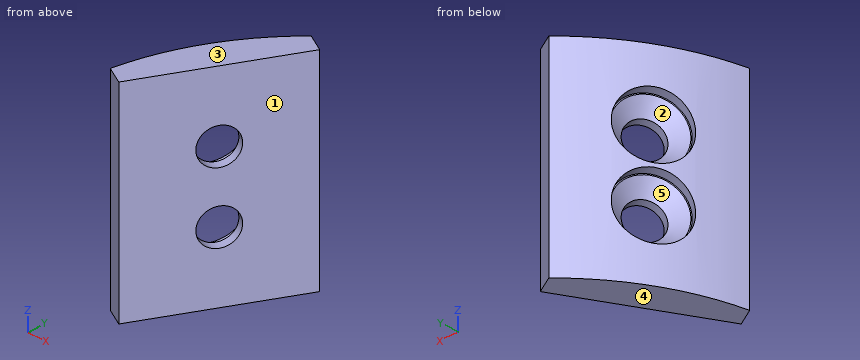
```python
from build123d import *

# Parameters (mm, degrees)
ESTRUSIONE_ESTRUSIONE1_DEPTH = 20
SCHIZZO3_R                   = 1.75
TAGLIO_ESTRUSIONE1_DEPTH     = 10.690610833
SCHIZZO3_3_R                 = 3.15
SCHIZZO3_3_R_2               = 1.75
TAGLIO_ESTRUSIONE2_DEPTH     = 1
SMUSSO2_SIZE                 = 1.3


with BuildPart() as part:
    # Schizzo2 → Estrusione-Estrusione1 (new body)
    with BuildSketch(Plane.XY):
        Polygon((-5.767949192, 11.990381057), (-7.5, 12.990381057), (-15, 0), (-13.267949192, -1), align=None)
        with BuildLine():
            Line((-15, 0), (-7.5, 12.990381057))
            ThreePointArc((-7.5, 12.990381057), (-12.285264352, 7.092900681), (-15, 0))
        make_face()
    extrude(amount=ESTRUSIONE_ESTRUSIONE1_DEPTH)

    # Schizzo3 → Taglio-Estrusione1 (cut, through all)
    with BuildSketch(Plane(origin=(-12.285264352, 7.092900681, 0), x_dir=(0, 0, 1), z_dir=(-0.866025404, 0.5, 0))):
        with Locations((6.666666667, 0)):
            Circle(SCHIZZO3_R)
        with Locations((13.333333333, 0)):
            Circle(SCHIZZO3_R)
    extrude(amount=-TAGLIO_ESTRUSIONE1_DEPTH, mode=Mode.SUBTRACT)

    # Schizzo3_3 → Taglio-Estrusione2 (cut)
    with BuildSketch(Plane(origin=(-12.285264352, 7.092900681, 0), x_dir=(0, 0, 1), z_dir=(-0.866025404, 0.5, 0))):
        with Locations((6.666666667, 0)):
            Circle(SCHIZZO3_3_R)
        with Locations((6.666666667, 0)):
            Circle(SCHIZZO3_3_R_2, mode=Mode.SUBTRACT)
        with Locations((13.333333333, 0)):
            Circle(SCHIZZO3_3_R)
        with Locations((13.333333333, 0)):
            Circle(SCHIZZO3_3_R_2, mode=Mode.SUBTRACT)
    extrude(amount=-TAGLIO_ESTRUSIONE2_DEPTH, mode=Mode.SUBTRACT)

    # Smusso2
    smusso2_edges = [part.edges().sort_by_distance(p)[0] for p in [
        (-11.419238948, 6.592900681, 4.916666667),
        (-11.419238948, 6.592900681, 11.583333333),
    ]]
    chamfer(smusso2_edges, length=SMUSSO2_SIZE)


solid = part.part
```
Here's how the part is built. I have some questions about the finished solid (model axes, mm). Face numbers are marked on the shaded views. A direction names the side the tool comes from. Give positions to 0.01 mm unless a question says otherwise; leave off trailing zeros. Order: outer loops, then holes, each group sorted by start corner. A loop starts at its lowest first (then second) coordinate and runs counter-clockwise, first axis right, second up. Notation, with made-up numbers: (16.25, 11.25) - (33.25, 11.25) arc R21 cw to (33.25, 25.25) - close; hole circle Ø9 at (-34.5, 9). An arc over 180 degrees is marked (long way). Answer as a JSON object with one key per item and string values. Group by question number.
Item 1: Please list where these lines run through material, in increasing order: probe 1 along Z at (x, y) = (-12, 7); probe 2 along Z at (x, y) = (-13.5, 4.5); probe 3 along X at (y, z) = (3.5, 5).
Item 2: If we mould it in two halves opening along Y, with no side actions, what happens to the marked faces 1, 2 and 3? For each: pulls with the +Y half, pulls with the -Y half, needs draft (parallel to the pull), parting line crosses it, or undercut.
Item 3: If we section it at A-A on z = 3: Please give me the cut outline in (x, y) (3 decimals), and give its area (3 significant figures).
Item 4: If we section it at B-B on x = -8.25: Please give me the cut outline in (y, z), and give its area (3 significant figures).
Item 5: For P1, Ø5, axis at x = -13, y = 4.5, coming from the -Z side; P2, Ø3, axis at y = 2.5, z = 2, coming from the +X side; P3, Ø3, axis at x = -8.5, z = 17.5, coming from the +Y side; P4, Ø4, axis at x = -14, z = 17.5, coming from the -Y side, each with a flat end and sliding along its axis, tell me the tip position at first contact or that it passes through.
Item 6: Which directions (+Z, -Z, +X, -X, +Y, -Y) give clear straight access to the entire face, cutting with the end or side of a thin tool? Please do the marked faces 4 and 5.
Result set:
{
 "1": {"probe 1": "0 to 3.52, 9.82 to 10.18, 16.48 to 20", "probe 2": "0 to 5.33, 8 to 12, 14.67 to 20", "probe 3": "-13.98 to -10.67"},
 "2": {"face 1": "pulls with the -Y half", "face 2": "undercut", "face 3": "needs draft"},
 "3": {"outline": "(-15, 0) - (-13.268, -1) - (-5.768, 11.99) - (-7.5, 12.99) arc R24.125 ccw to start", "area": "42.0 mm²"},
 "4": {"outline": "(7.69, 0) - (12.29, 0) - (12.29, 20) - (7.69, 20) - close", "area": "91.9 mm²"},
 "5": {"P1": "z = 0", "P2": "x = -10.38", "P3": "y = 12.99", "P4": "y = -1"},
 "6": {"face 4": "-Z, +X, -X, +Y, -Y", "face 5": "none"}
}
